from build123d import *

# Parameters (mm, degrees)
F1_R          = 63.75
F2_DEPTH      = 10
F3_R          = 6.35
F4_DEPTH      = 14
F5_R          = 6.5
F6_DEPTH      = 10.001
F6_DEPTH_BACK = 14.001
F7_SIZE       = 2


with BuildPart() as f2:
    # F1 (on Front) → F2 (new body)
    with BuildSketch(Plane.XZ):
        Circle(F1_R)
    extrude(amount=-F2_DEPTH)

    # F3 (on Front) → F4 (join)
    with BuildSketch(Plane.XZ):
        with BuildLine():
            ThreePointArc((-22.7778931025, -22.1185461957), (0, -18.5), (22.7778931025, -22.1185461957))
            ThreePointArc((22.7778931025, -22.1185461957), (0, 31.75), (-22.7778931025, -22.1185461957))
        make_face()
        with Locations((0, -53.5)):
            Circle(F3_R)
    extrude(amount=F4_DEPTH)

    # F5 (on Front) → F6 (cut, two sides)
    with BuildSketch(Plane.XZ) as f6_sk:
        Circle(F5_R)
    extrude(amount=-F6_DEPTH, mode=Mode.SUBTRACT)
    extrude(f6_sk.sketch, amount=F6_DEPTH_BACK, mode=Mode.SUBTRACT)

    # F7
    f7_edges = [f2.edges().sort_by_distance(p)[0] for p in [
        (-6.5, 10, 0),
    ]]
    chamfer(f7_edges, length=F7_SIZE)


solid = f2.part
Input: part model. Units: mm. Frame: model coordinates. A direction names the side the tool comes from. Round coordinates to 2 decimals unless told otherwise and drop trailing zeros. Order: outer loops, then holes, each group sorted by start corner. A loop starts at its lowest first (then second) coordinate and runs counter-clockwise, first axis right, second up. Notation, with made-up numbers: (19.5, 31) - (73.5, 31) arc R20 ccw to (73.5, 58) - close; hole circle Ø10 at (-15.75, -10). An arc over 180 degrees is marked (long way). Answer as a JSON object with one key per item and string values. Group by question number.
(1) Cut plane A-A (z = 0). Return loops of the section in (x, y), then the cut area to 3 significant figures.
(2) Pin query (flat end, axial travel): P1, Ø6, axis at y = -1.5, z = -37, coming from the -X side; P2, Ø4, axis at x = -14.5, y = 3.5, coming from the -Z side; P3, Ø11.5, axis at x = 0, z = 0, coming from the +Y side; P4, Ø4, axis at x = -34.5, z = -44, coming from the -Y side. Return the tip coordinate at first contact, or that it passes through.
(3) Material intervals for probe 1 along Z at (x, y) = (0, -0.75); probe 2 along X at (y, z) = (-4.5, 0); probe 3 along Y at (x, z) = (30, 53), sorted ascending. Write a range as from..to.
(4) Cut plane B-B (x = 0). Return loops of the section in (y, z), then the cut area to 3 significant figures.
(5) Cut plane C-C (y = -7). Return loops of the section in (x, z), then the cut area to 3 significant figures.
(6) Draft query along X for faces 1 (the face through (-5.158, -3.154, -3.955)), 2 (the face through (0, -14, -53)), 3 (the face through (-0.3, -6.9, -18.5)), 4 (the face through (-13.82, 4.93, -62.234)). Return one class per face: released by +X, released by -X, zero draft, split by the parting line, or undercut.
(7) Cut plane D-D (z = -53.5). Return loops of the section in (x, y).
(8) Reachability of faces 5 (the face through (1.041, -6.902, 31.733)), 6 (the face through (-8, -14, 5)) from +Z, -Z, +X, -X, +Y, -Y: full face, straight path, thin tool, end or side. Return the list, or none.
Here are the results:
{
 "1": {"outline": "(-63.75, 0) - (-31.75, 0) - (-31.75, -14) - (-6.5, -14) - (-6.5, 8) - (-8.5, 10) - (-63.75, 10) - close; (6.5, -14) - (31.75, -14) - (31.75, 0) - (63.75, 0) - (63.75, 10) - (8.5, 10) - (6.5, 8) - close", "area": "1,850 mm^2"},
 "2": {"P1": "stops at x = -53.67", "P2": "stops at z = -62.51", "P3": "passes through", "P4": "stops at y = 0"},
 "3": {"probe 1": "z = -59.85..-47.15, -18.5..-6.5, 6.5..31.75", "probe 2": "x = -31.75..-6.5, 6.5..31.75", "probe 3": "y = 0..10"},
 "4": {"outline": "(-14, -59.85) - (0, -59.85) - (0, -63.75) - (10, -63.75) - (10, -8.5) - (8, -6.5) - (-14, -6.5) - (-14, -18.5) - (0, -18.5) - (0, -47.15) - (-14, -47.15) - close; (-14, 6.5) - (8, 6.5) - (10, 8.5) - (10, 63.75) - (0, 63.75) - (0, 31.75) - (-14, 31.75) - close", "area": "1,840 mm^2"},
 "5": {"outline": "(-22.78, -22.12) arc R73.5 cw to (22.78, -22.12) arc R31.75 ccw (long way) to start; circle Ø12.7 at (0, -53.5); hole circle Ø13 at (0, 0)", "area": "2,750 mm^2"},
 "6": {"face 1": "undercut", "face 2": "zero draft", "face 3": "undercut", "face 4": "split by the parting line"},
 "7": {"outline": "(-34.67, 0) - (-6.35, 0) - (-6.35, -14) - (6.35, -14) - (6.35, 0) - (34.67, 0) - (34.67, 10) - (-34.67, 10) - close"},
 "8": {"face 5": "-Y", "face 6": "+Z, -Z, +X, -X, -Y"}
}
